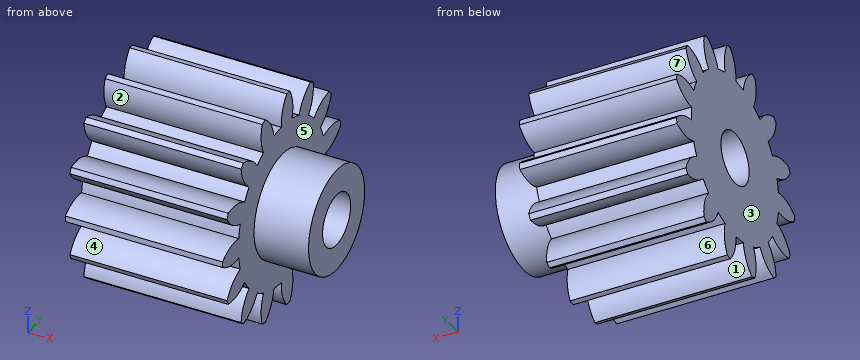
```python
from build123d import *

# Parameters (mm, degrees)
SPUR_START             = -77.326171545
SPUR_GEAR_AI_OUTLINE_R = 1.5875
SPUR_GEAR_AI_DEPTH     = 9.525
SKETCH1_R              = 3.175
SKETCH1_R_2            = 1.5875
BOSS_EXTRUDE1_DEPTH    = 3.302


# Read off the part's stored shape, not the designer's step: spur gear_ai
with BuildPart() as part:
    # spur gear_ai outline → spur gear_ai (new body)
    with BuildSketch(Plane.YZ.offset(SPUR_START)):
        with BuildLine():
            ThreePointArc((25.700043696, 22.871890839), (25.806291245, 23.014153087), (25.908758385, 23.159161964))
            ThreePointArc((25.908758385, 23.159161964), (25.44365934, 24.001503635), (24.683177407, 24.591015164))
            ThreePointArc((24.683177407, 24.591015164), (24.869844856, 24.966591507), (25.024047568, 25.356622082))
            ThreePointArc((25.024047568, 25.356622082), (25.971001747, 25.185934076), (26.908195608, 25.40393472))
            ThreePointArc((26.908195608, 25.40393472), (26.947394305, 25.577112523), (26.982022272, 25.751261864))
            ThreePointArc((26.982022272, 25.751261864), (26.214521927, 26.331606447), (25.280011171, 26.560836158))
            ThreePointArc((25.280011171, 26.560836158), (25.297779711, 26.979866711), (25.280011171, 27.398897265))
            ThreePointArc((25.280011171, 27.398897265), (26.214521927, 27.628126976), (26.982022272, 28.208471559))
            ThreePointArc((26.982022272, 28.208471559), (26.947394305, 28.3826209), (26.908195608, 28.555798703))
            ThreePointArc((26.908195608, 28.555798703), (25.971001747, 28.773799347), (25.024047568, 28.60311134))
            ThreePointArc((25.024047568, 28.60311134), (24.869844856, 28.993141915), (24.683177407, 29.368718258))
            ThreePointArc((24.683177407, 29.368718258), (25.44365934, 29.958229787), (25.908758385, 30.800571458))
            ThreePointArc((25.908758385, 30.800571458), (25.806291245, 30.945580335), (25.700043696, 31.087842584))
            ThreePointArc((25.700043696, 31.087842584), (24.755205651, 30.905804997), (23.959545029, 30.36471278))
            ThreePointArc((23.959545029, 30.36471278), (23.660034115, 30.658303547), (23.336744253, 30.925485117))
            ThreePointArc((23.336744253, 30.925485117), (23.791703129, 31.773346565), (23.873981026, 32.732036797))
            ThreePointArc((23.873981026, 32.732036797), (23.721392211, 32.822831857), (23.566466975, 32.909580117))
            ThreePointArc((23.566466975, 32.909580117), (22.777355829, 32.358980252), (22.270565713, 31.541043584))
            ThreePointArc((22.270565713, 31.541043584), (21.877534755, 31.687430032), (21.473522236, 31.800018709))
            ThreePointArc((21.473522236, 31.800018709), (21.544291531, 32.759627129), (21.229521683, 33.668899671))
            ThreePointArc((21.229521683, 33.668899671), (21.053195187, 33.689781624), (20.876380246, 33.706016332))
            ThreePointArc((20.876380246, 33.706016332), (20.379440483, 32.882057908), (20.249149489, 31.92870547))
            ThreePointArc((20.249149489, 31.92870547), (19.83055711, 31.902576052), (19.415679368, 31.84110423))
            ThreePointArc((19.415679368, 31.84110423), (19.090022428, 32.746534609), (18.432631403, 33.449167979))
            ThreePointArc((18.432631403, 33.449167979), (18.263055677, 33.396526145), (18.09492394, 33.339440173))
            ThreePointArc((18.09492394, 33.339440173), (17.976080961, 32.384593086), (18.244817586, 31.460668176))
            ThreePointArc((18.244817586, 31.460668176), (17.873042211, 31.266540906), (17.519035377, 31.041637622))
            ThreePointArc((17.519035377, 31.041637622), (16.853261246, 31.736332821), (15.966917922, 32.110835325))
            ThreePointArc((15.966917922, 32.110835325), (15.833414151, 31.993771955), (15.703037123, 31.873235987))
            ThreePointArc((15.703037123, 31.873235987), (15.982839958, 30.952601973), (16.604137198, 30.217859601))
            ThreePointArc((16.604137198, 30.217859601), (16.343462167, 29.889300848), (16.111537238, 29.539853923))
            ThreePointArc((16.111537238, 29.539853923), (15.220764312, 29.903694832), (14.258725503, 29.885311585))
            ThreePointArc((14.258725503, 29.885311585), (14.184377702, 29.724068), (14.114298755, 29.560923799))
            ThreePointArc((14.114298755, 29.560923799), (14.744366952, 28.833688843), (15.610796869, 28.41517264))
            ThreePointArc((15.610796869, 28.41517264), (15.506295264, 28.008993196), (15.436554167, 27.595425178))
            ThreePointArc((15.436554167, 27.595425178), (14.474805177, 27.565500398), (13.603416133, 27.157410031))
            ThreePointArc((13.603416133, 27.157410031), (13.601079711, 26.979866712), (13.603416133, 26.802323392))
            ThreePointArc((13.603416133, 26.802323392), (14.474805177, 26.394233025), (15.436554167, 26.364308244))
            ThreePointArc((15.436554167, 26.364308244), (15.506295264, 25.950740226), (15.610796869, 25.544560783))
            ThreePointArc((15.610796869, 25.544560783), (14.744366952, 25.12604458), (14.114298755, 24.398809624))
            ThreePointArc((14.114298755, 24.398809624), (14.184377702, 24.235665423), (14.258725503, 24.074421838))
            ThreePointArc((14.258725503, 24.074421838), (15.220764312, 24.056038591), (16.111537238, 24.4198795))
            ThreePointArc((16.111537238, 24.4198795), (16.343462167, 24.070432575), (16.604137198, 23.741873821))
            ThreePointArc((16.604137198, 23.741873821), (15.982839958, 23.007131449), (15.703037123, 22.086497436))
            ThreePointArc((15.703037123, 22.086497436), (15.833414152, 21.965961467), (15.966917922, 21.848898097))
            ThreePointArc((15.966917922, 21.848898097), (16.853261246, 22.223400602), (17.519035377, 22.918095801))
            ThreePointArc((17.519035377, 22.918095801), (17.873042211, 22.693192517), (18.244817586, 22.499065247))
            ThreePointArc((18.244817586, 22.499065247), (17.976080961, 21.575140337), (18.09492394, 20.62029325))
            ThreePointArc((18.09492394, 20.62029325), (18.263055677, 20.563207278), (18.432631403, 20.510565444))
            ThreePointArc((18.432631403, 20.510565444), (19.090022428, 21.213198814), (19.415679368, 22.118629192))
            ThreePointArc((19.415679368, 22.118629192), (19.83055711, 22.057157371), (20.249149489, 22.031027953))
            ThreePointArc((20.249149489, 22.031027953), (20.379440483, 21.077675515), (20.876380246, 20.253717091))
            ThreePointArc((20.876380246, 20.253717091), (21.053195187, 20.269951799), (21.229521683, 20.290833751))
            ThreePointArc((21.229521683, 20.290833751), (21.544291531, 21.200106294), (21.473522236, 22.159714714))
            ThreePointArc((21.473522236, 22.159714714), (21.877534755, 22.272303391), (22.270565713, 22.418689838))
            ThreePointArc((22.270565713, 22.418689838), (22.777355829, 21.600753171), (23.566466975, 21.050153306))
            ThreePointArc((23.566466975, 21.050153306), (23.721392211, 21.136901565), (23.873981026, 21.227696625))
            ThreePointArc((23.873981026, 21.227696625), (23.791703129, 22.186386858), (23.336744253, 23.034248306))
            ThreePointArc((23.336744253, 23.034248306), (23.660034115, 23.301429876), (23.959545029, 23.595020643))
            ThreePointArc((23.959545029, 23.595020643), (24.755205651, 23.053928425), (25.700043696, 22.871890839))
        make_face()
        with Locations((20.347954711, 26.979866711)):
            Circle(SPUR_GEAR_AI_OUTLINE_R, mode=Mode.SUBTRACT)
    extrude(amount=SPUR_GEAR_AI_DEPTH)

    # Sketch1 → Boss-Extrude1 (add)
    with BuildSketch(Plane(origin=(-67.801171545, 0, 0), x_dir=(0, 0, -1), z_dir=(1, 0, 0))):
        with Locations(Location((-26.979866711, 20.347954711, 0), (0, 0, 180))):
            Circle(SKETCH1_R)
        with Locations((-26.979866711, 20.347954711)):
            Circle(SKETCH1_R_2, mode=Mode.SUBTRACT)
    extrude(amount=BOSS_EXTRUDE1_DEPTH)


solid = part.part
```
Input: part model. Units: mm. Frame: model coordinates. Face numbers are marked on the shaded views. A direction names the side the tool comes from. Coordinates: 2 decimals unless noted, no trailing zeros. Write each loop counter-clockwise with the first axis right and the second up, starting at its lowest first coordinate (ties: lowest second). Pieces come first, ordered by that corner, then holes. Notation, with made-up numbers: (25.25, -25) -> (58.25, -25) arc R29 ccw to (58.25, 5) -> close; hole circle Ø8 at (48, 11.5). An arc over 180 degrees is marked (long way). Write each question's results on one line, items separated by ' | '.
Item 1: Set-up query: the marked faces 4, 5, 6 and 7. Return all of +Z, -Z, +X, -X, +Y, -Y with unobstructed straight access to the full face (end or side cutting, diameter ignored); none if empty.
Conclusion:
face 4: +X, -X, -Y | face 5: +X | face 6: +X, -X | face 7: +X, -X, +Y
Item 2: Mould query, pull axis Z, two halves, no side actions, for the marked faces 1, 2 and 3. Classes: +Z half, -Z half, draft (parallel to the pull), parting line (faces both ways), or undercut.
Conclusion:
face 1: -Z half | face 2: undercut | face 3: draft
Item 3: Section query A-A on y = 15. Return loops of the section in (x, z).
Conclusion:
outline: (-77.33, 24.03) -> (-67.8, 24.03) -> (-67.8, 25.3) -> (-77.33, 25.3) -> close; (-77.33, 26.33) -> (-67.8, 26.33) -> (-67.8, 27.63) -> (-77.33, 27.63) -> close; (-77.33, 28.66) -> (-67.8, 28.66) -> (-67.8, 29.93) -> (-77.33, 29.93) -> close
Item 4: Material intervals for probe 1 along Y at (x, z) = (-66, 27); probe 2 along Z at (x, y) = (-74.5, 25.5); probe 3 along Y at (x, z) = (-69.75, 27), sorted ascending.
Conclusion:
probe 1: y = 17.17 to 18.76, 21.94 to 23.52 | probe 2: z = 22.88 to 23.93, 25.22 to 26.54, 27.42 to 28.74, 30.03 to 31.08 | probe 3: y = 13.6 to 18.76, 21.94 to 25.3
Item 5: Pin query (flat end, axial travel): pin 1 Ø3 at (x, y) = (-73.5, 15.5) entering from -Z. Return the tip coordinate at first contact, or that it passes through.
Conclusion:
pin 1: stops at z = 21.85
Item 6: Section query B-B on z = 32.5. Return loops of the section in (x, y).
Conclusion:
outline: (-77.33, 17.97) -> (-67.8, 17.97) -> (-67.8, 19.22) -> (-77.33, 19.22) -> close; (-77.33, 20.28) -> (-67.8, 20.28) -> (-67.8, 21.56) -> (-77.33, 21.56) -> close; (-77.33, 22.92) -> (-67.8, 22.92) -> (-67.8, 23.89) -> (-77.33, 23.89) -> close
